from build123d import *

# Parameters (mm, degrees)
SKETCH2_R           = 30
BOSS_EXTRUDE2_DEPTH = 130
SKETCH3_R           = 22
CUT_EXTRUDE1_DEPTH  = 131
CUT_EXTRUDE2_REACH  = 62
SKETCH4_W           = 30
SKETCH4_H           = 140
SKETCH5_W           = 130
SKETCH5_H           = 40
BOSS_EXTRUDE3_DEPTH = 7.63932
SKETCH6_W           = 130
SKETCH6_H           = 60
BOSS_EXTRUDE4_DEPTH = 10


with BuildPart() as part:
    # Sketch2 → Boss-Extrude2 (new body)
    with BuildSketch(Plane.XY):
        Circle(SKETCH2_R)
    extrude(amount=BOSS_EXTRUDE2_DEPTH)

    # Sketch3 → Cut-Extrude1 (cut, through all)
    with BuildSketch(Plane.XY.offset(130)):
        Circle(SKETCH3_R)
    extrude(amount=-CUT_EXTRUDE1_DEPTH, mode=Mode.SUBTRACT)

    # Sketch4 → Cut-Extrude2 (cut, up to next)
    with BuildSketch(Plane(origin=(0, -30, 0), x_dir=(1, 0, 0), z_dir=(0, 1, 0)), mode=Mode.PRIVATE) as cut_extrude2_sk1:
        with Locations((0, -70)):
            Rectangle(SKETCH4_W, SKETCH4_H)
    cut_extrude2_tool1 = extrude(cut_extrude2_sk1.sketch, amount=CUT_EXTRUDE2_REACH, mode=Mode.PRIVATE) & part.part
    add(cut_extrude2_tool1.solids().sort_by_distance((0, -30, 70))[0], mode=Mode.SUBTRACT)

    # Sketch5 → Boss-Extrude3 (add)
    with BuildSketch(Plane(origin=(-30, 0, 0), x_dir=(0, 0, -1), z_dir=(1, 0, 0))):
        with Locations((-65, 0)):
            Rectangle(SKETCH5_W, SKETCH5_H)
    extrude(amount=BOSS_EXTRUDE3_DEPTH)

    # Sketch6 → Boss-Extrude4 (add)
    with BuildSketch(Plane.ZY.offset(30)):
        with Locations((65, 0)):
            Rectangle(SKETCH6_W, SKETCH6_H)
    extrude(amount=BOSS_EXTRUDE4_DEPTH)


solid = part.part
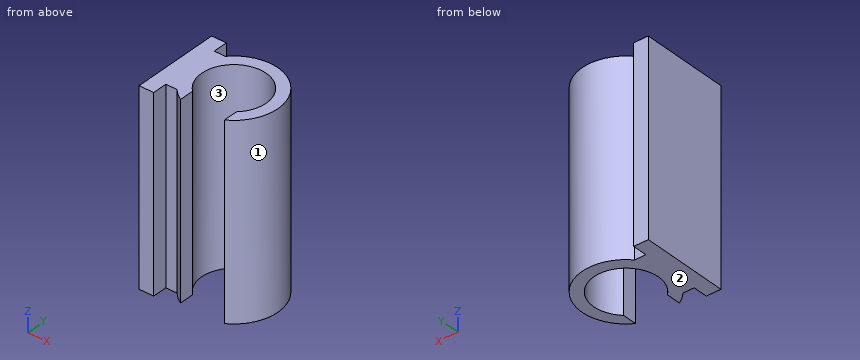
Read the model definition and answer for the solid it produces. Units are mm, in the model's axes. Face numbers are marked on the shaded views. Round coordinates to 2 decimals unless told otherwise and drop trailing zeros. Order: outer loops, then holes, each group sorted by start corner. A loop starts at its lowest first (then second) coordinate and runs counter-clockwise, first axis right, second up.
1) The mould has two halves that part along Y. Classify the marked faces 1, 2 and 3: released by +Y, released by -Y, zero draft, split by the parting line, or undercut.
2) Straight lines are drawn through the part: L1, parallel to X at y = 0, z = 61.5; L2, parallel to X at y = -25, z = 65.5; L3, parallel to X at y = -7, z = 113. For each, find the intervals that lie inside material, in ascending order.
3) Flat-ended cylindrical pins translate along their axes: pin 1 (5 mm diameter, centred on y = -25.5, z = 48, fed in from +X); pin 2 (4 mm diameter, centred on x = -26.5, z = 91.5, fed in from +Y); pin 3 (11 mm diameter, centred on y = 25.5, z = 70.5, fed in from +X). Find the tip coordinate at first contact, or state that the pin passes through.
4) The part is cut by section C-C on y = -23. Write down the section's boundary in (x, z), plus the area to 3 significant figures.
5) The part is cut by section D-D on x = 19.5. Write down the section's boundary in (y, z), plus the area to 3 significant figures.
6) The part is cut by section B-B on y = 0. Write down the section's boundary in (x, z), plus the area to 3 significant figures.
7) The part is cut by section A-A on z = 92. Write down the section's boundary in (x, y), plus the area to 3 significant figures.
Resolved:
1. face 1: split by the parting line
1. face 2: zero draft
1. face 3: undercut
2. L1: x = -40 to -22, 22 to 30
2. L2: x = -40 to -30, -16.58 to -15, 15 to 16.58
2. L3: x = -40 to -20.86, 20.86 to 29.17
3. pin 1: stops at x = 19.26
3. pin 2: stops at y = 20
3. pin 3: stops at x = 22.36
4. outline: (-40, 0) - (-30, 0) - (-30, 130) - (-40, 130) - close; (-19.26, 0) - (-15, 0) - (-15, 130) - (-19.26, 130) - close; (15, 0) - (19.26, 0) - (19.26, 130) - (15, 130) - close
4. area: 2,410 mm2
5. outline: (-22.8, 0) - (-10.19, 0) - (-10.19, 130) - (-22.8, 130) - close; (10.19, 0) - (22.8, 0) - (22.8, 130) - (10.19, 130) - close
5. area: 3,280 mm2
6. outline: (-40, 0) - (-22, 0) - (-22, 130) - (-40, 130) - close; (22, 0) - (30, 0) - (30, 130) - (22, 130) - close
6. area: 3,380 mm2
7. outline: (-40, -30) - (-30, -30) - (-30, -20) - (-22.36, -20) arc R30 ccw to (-15, -25.98) - (-15, -16.09) arc R22 cw (long way) to (15, -16.09) - (15, -25.98) arc R30 ccw (long way) to (-22.36, 20) - (-30, 20) - (-30, 30) - (-40, 30) - close
7. area: 1,750 mm2
